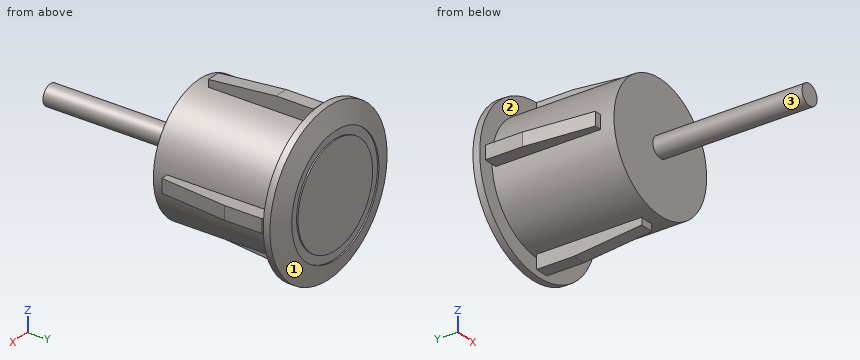
```python
from build123d import *
from OCP.BRepFilletAPI import BRepFilletAPI_MakeChamfer

# Parameters (mm, degrees)
SKETCH_1_R          = 9.3
EXTRUDE_1_DEPTH     = 20
SKETCH_2_R          = 11.75
EXTRUDE_2_DEPTH     = 2
CHAMFER_1_SIZE      = 1
CHAMFER_1_SIZE2     = 3
SKETCH_3_R          = 1.5
EXTRUDE_3_DEPTH     = 22
EXTRUDE_START       = -2
SKETCH_4_W          = 2
SKETCH_4_H          = 4
SKETCH_4_W_2        = 4
SKETCH_4_H_2        = 2
EXTRUDE_4_DEPTH     = 15.5
CHAMFER_2_SIZE      = 10
CHAMFER_2_SIZE2     = 1
SKETCH_5_R          = 8.75
SKETCH_5_R_2        = 7.5
CUT_EXTRUDE_1_DEPTH = 0.2


with BuildPart() as part:
    # 草图1 → 凸台-拉伸1 (new body)
    with BuildSketch(Plane(origin=(0, 0, 0), x_dir=(1, 0, 0), z_dir=(0, 1, 0))):
        with Locations(Location((0, 0, 0), (0, 0, 270))):
            Circle(SKETCH_1_R)
    extrude(amount=EXTRUDE_1_DEPTH)

    # 草图2 → 凸台-拉伸2 (add)
    with BuildSketch(Plane(origin=(0, 20, 0), x_dir=(1, 0, 0), z_dir=(0, 1, 0))):
        with Locations(Location((0, 0, 0), (0, 0, 270))):
            Circle(SKETCH_2_R)
    extrude(amount=-EXTRUDE_2_DEPTH)

    # 倒角1
    chamfer_1_edges = [part.edges().sort_by_distance(p)[0] for p in [
        (0, 20, -11.75),
    ]]
    chamfer_1_side = [part.faces().sort_by_distance(p)[0] for p in [
        (0, 19, -11.75),
    ]]
    chamfer(chamfer_1_edges, length=CHAMFER_1_SIZE, length2=CHAMFER_1_SIZE2, reference=chamfer_1_side[0])

    # 草图3 → 凸台-拉伸3 (add)
    with BuildSketch(Plane.XZ):
        with Locations(Location((0, 0, 0), (0, 0, 90))):
            Circle(SKETCH_3_R)
    extrude(amount=EXTRUDE_3_DEPTH)

    # 草图4 → 凸台-拉伸4 (add)
    with BuildSketch(Plane.XZ.offset(EXTRUDE_START)):
        with Locations((0, 9.3)):
            Rectangle(SKETCH_4_W, SKETCH_4_H)
        with Locations((0, -9.3)):
            Rectangle(SKETCH_4_W, SKETCH_4_H)
        with Locations((-9.3, 0)):
            Rectangle(SKETCH_4_W_2, SKETCH_4_H_2)
        with Locations((9.3, 0)):
            Rectangle(SKETCH_4_W_2, SKETCH_4_H_2)
    extrude(amount=-EXTRUDE_4_DEPTH)

    # 倒角2: one chamfer whose edges measure the first distance from different faces: ONE call of the kernel's chamfer builder (chamfer() names one face for all edges)
    chamfer_2_edges_1 = [part.edges().sort_by_distance(p)[0] for p in [
        (0, 2, 11.3),
    ]]
    chamfer_2_side_1 = [part.faces().sort_by_distance(p)[0] for p in [
        (0, 9.75, 11.3),
    ]]
    chamfer_2_edges_2 = [part.edges().sort_by_distance(p)[0] for p in [
        (0, 2, -11.3),
    ]]
    chamfer_2_side_2 = [part.faces().sort_by_distance(p)[0] for p in [
        (0, 9.75, -11.3),
    ]]
    chamfer_2_edges_3 = [part.edges().sort_by_distance(p)[0] for p in [
        (-11.3, 2, 0),
    ]]
    chamfer_2_side_3 = [part.faces().sort_by_distance(p)[0] for p in [
        (-11.3, 9.75, 0),
    ]]
    chamfer_2_edges_4 = [part.edges().sort_by_distance(p)[0] for p in [
        (11.3, 2, 0),
    ]]
    chamfer_2_side_4 = [part.faces().sort_by_distance(p)[0] for p in [
        (11.3, 9.75, 0),
    ]]
    chamfer_2 = BRepFilletAPI_MakeChamfer(part.part.solid().wrapped)
    for e in chamfer_2_edges_1:
        chamfer_2.Add(CHAMFER_2_SIZE, CHAMFER_2_SIZE2, e.wrapped, chamfer_2_side_1[0].wrapped)  # the first distance lies on this face
    for e in chamfer_2_edges_2:
        chamfer_2.Add(CHAMFER_2_SIZE, CHAMFER_2_SIZE2, e.wrapped, chamfer_2_side_2[0].wrapped)  # the first distance lies on this face
    for e in chamfer_2_edges_3:
        chamfer_2.Add(CHAMFER_2_SIZE, CHAMFER_2_SIZE2, e.wrapped, chamfer_2_side_3[0].wrapped)  # the first distance lies on this face
    for e in chamfer_2_edges_4:
        chamfer_2.Add(CHAMFER_2_SIZE, CHAMFER_2_SIZE2, e.wrapped, chamfer_2_side_4[0].wrapped)  # the first distance lies on this face
    add(Compound.cast(chamfer_2.Shape()), mode=Mode.REPLACE)

    # 草图5 → 切除-拉伸1 (cut)
    with BuildSketch(Plane(origin=(0, 20, 0), x_dir=(1, 0, 0), z_dir=(0, 1, 0))):
        with Locations(Location((0, 0, 0), (0, 0, 270))):
            Circle(SKETCH_5_R)
        with Locations(Location((0, 0, 0), (0, 0, 270))):
            Circle(SKETCH_5_R_2, mode=Mode.SUBTRACT)
    extrude(amount=-CUT_EXTRUDE_1_DEPTH, mode=Mode.SUBTRACT)


solid = part.part
```
Check sheet for the modelled part. Datum: model origin and axes. Units: mm. Face numbers are marked on the shaded views. A direction names the side the tool comes from. Coordinates: 2 decimals unless noted, no trailing zeros. Order: outer loops, then holes, each group sorted by start corner. A loop starts at its lowest first (then second) coordinate and runs counter-clockwise, first axis right, second up. Notation, with made-up numbers: M 31,77.5 L 67,77.5 A15 cw 67,90.5 Z; hole C 33,-36.5 d1. An arc over 180 degrees is marked long. One line per question, with ' | ' between items. Start each with the question number.
Item 1: Access from +Z, -Z, +X, -X, +Y, -Y to the whole of each face (thin tool, end or side, straight path). Record for the marked faces 1, 2 and 3.
Item 2: Sectioned sample at D-D on y = 7. Record the cut outline in (x, z).
Item 3: Gauge pin test, flat ends, axial feed: P1, Ø4, axis at x = 9, z = -0.5, coming from the +Y side; P2, Ø0.6, axis at y = 15, z = 0, coming from the +X side; P3, Ø1, axis at x = 10.5, z = 0.5, coming from the +Y side; P4, Ø0.6, axis at x = 0.5, z = 10, coming from the +Y side. Record the tip position at first contact, or that the pin passes through.
Item 4: Material ranges on line 1 (Y direction, x = 2.25, z = -7.5); line 2 (Y direction, x = 0.5, z = -10); line 3 (Y direction, x = 1.25, z = -5.5), recorded low to high.
Item 5: Sectioned sample at B-B on y = 13. Record the cut outline in (x, z).
Answer below:
1) face 1: +Y | face 2: none | face 3: -Y
2) outline: M -10.8,-1 L -9.25,-1 A9.3 ccw -1,-9.25 L -1,-10.8 L 1,-10.8 L 1,-9.25 A9.3 ccw 9.25,-1 L 10.8,-1 L 10.8,1 L 9.25,1 A9.3 ccw 1,9.25 L 1,10.8 L -1,10.8 L -1,9.25 A9.3 ccw -9.25,1 L -10.8,1 Z
3) P1: stops at y = 20 | P2: stops at x = 11.3 | P3: stops at y = 19.58 | P4: stops at y = 19.68
4) line 1: y = 0 to 19.8 | line 2: y = 2 to 17.5, 18 to 19.58 | line 3: y = 0 to 20
5) outline: M -11.3,-1 L -9.25,-1 A9.3 ccw -1,-9.25 L -1,-11.3 L 1,-11.3 L 1,-9.25 A9.3 ccw 9.25,-1 L 11.3,-1 L 11.3,1 L 9.25,1 A9.3 ccw 1,9.25 L 1,11.3 L -1,11.3 L -1,9.25 A9.3 ccw -9.25,1 L -11.3,1 Z
